Can you work these out from the drawing? Everything is in mm from the part's minimum corner. A direction names the side the tool comes from. Coordinates: 2 decimals unless noted, no trailing zeros. Order: outer loops, then holes, each group sorted by start corner. A loop starts at its lowest first (then second) coordinate and runs counter-clockwise, first axis right, second up. Notation, with made-up numbers: (84, -12.5) -> (122, -12.5) arc R18 cw to (122, 4.5) -> close; hole circle Ø7 at (43.25, 81). An arc over 180 degrees is marked (long way). Put each result on its own line as item: value. Start each with the question number.
Q1. Will these pins go through, and if not, where does the flat tip stop? pin 1 (4 mm diameter, centred on y = 5, z = 3.5, fed in from +X); pin 2 (12 mm diameter, centred on x = 4.5, z = 6, fed in from +Y); pin 3 (2 mm diameter, centred on x = 6.5, y = 6, fed in from -Z).
Q2. If we section it at B-B (x = 8.25): Please give me the cut outline in (y, z).
Q3. If we section it at D-D (x = 18.25): Please give me the cut outline in (y, z) (1 decimal).
Q4. Please list where these lines run through material, in increasing order: line 1 along Y through (x, z) = (1.75, 4.5); line 2 along X through (y, z) = (1.6, 8.5) (1 decimal); line 3 along Z through (x, y) = (7, 5.75).
Q5. For the marked faces 1 and 2, which set-ups out of +Z, -Z, +X, -X, +Y, -Y let a thin tool reach every point of the face, with its end or its side?
Q6. If we section it at A-A (z = 10.75): Please give me the cut outline in (x, y), and give its area (3 significant figures).
Q7. We'd pull the mould along Z, two halves only. Please class the marked faces 3, 4 and 5: +Z half, -Z half, draft (parallel to the pull), parting line (faces both ways), or undercut.
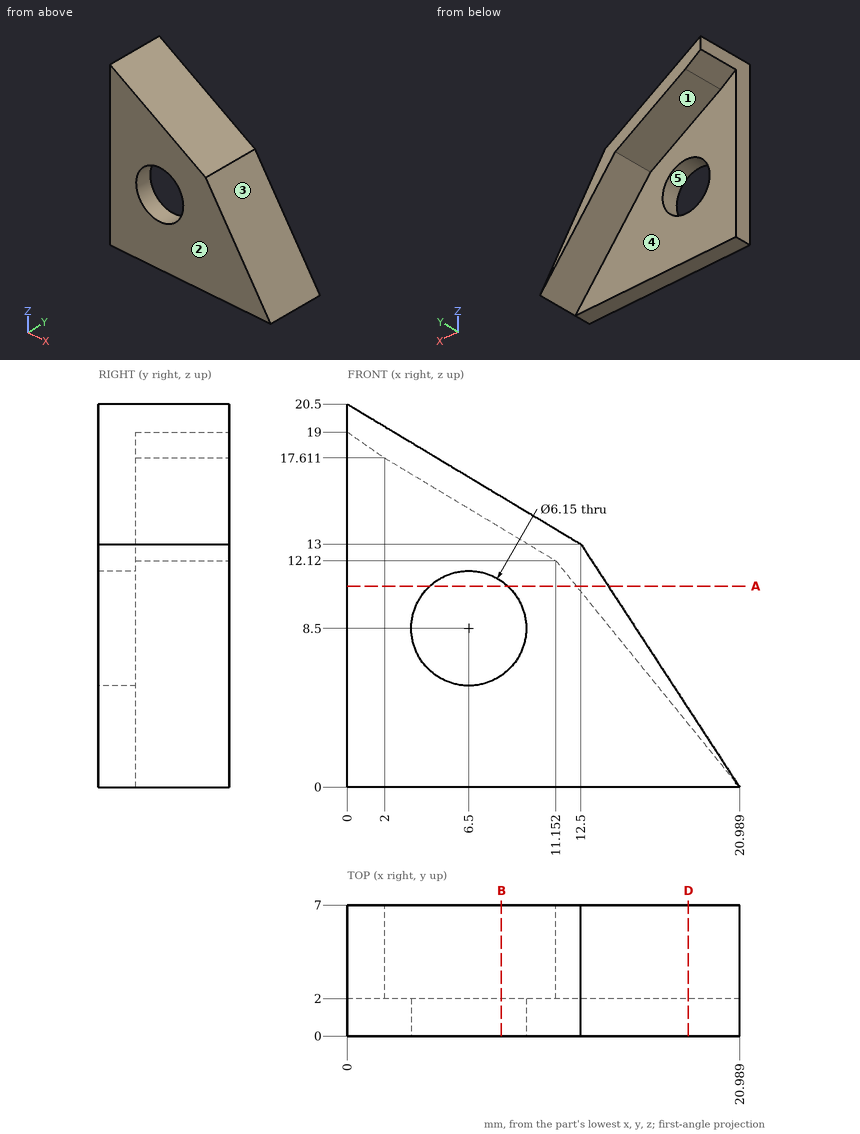
The answers:
1. pin 1: x = 20.01
1. pin 2: y = 2
1. pin 3: z = 14.31
2. outline: (0, 0) -> (2, 0) -> (2, 5.97) -> (0, 5.97) -> close; (0, 11.03) -> (2, 11.03) -> (2, 13.86) -> (7, 13.86) -> (7, 15.55) -> (0, 15.55) -> close
3. outline: (0, 0) -> (2, 0) -> (2, 3.4) -> (7, 3.4) -> (7, 4.2) -> (0, 4.2) -> close
4. line 1: 0 to 2
4. line 2: 0 to 3.4, 9.6 to 15.4
4. line 3: 14.61 to 16.3
5. face 1: -Z, -X, +Y
5. face 2: +Z, -Z, +X, -X, -Y
6. outline: (0, 0) -> (4.4, 0) -> (4.4, 2) -> (0, 2) -> close; (8.6, 0) -> (13.97, 0) -> (13.97, 7) -> (12.26, 7) -> (12.26, 2) -> (8.6, 2) -> close
6. area: 28.1 mm^2
7. face 3: +Z half
7. face 4: draft
7. face 5: undercut
